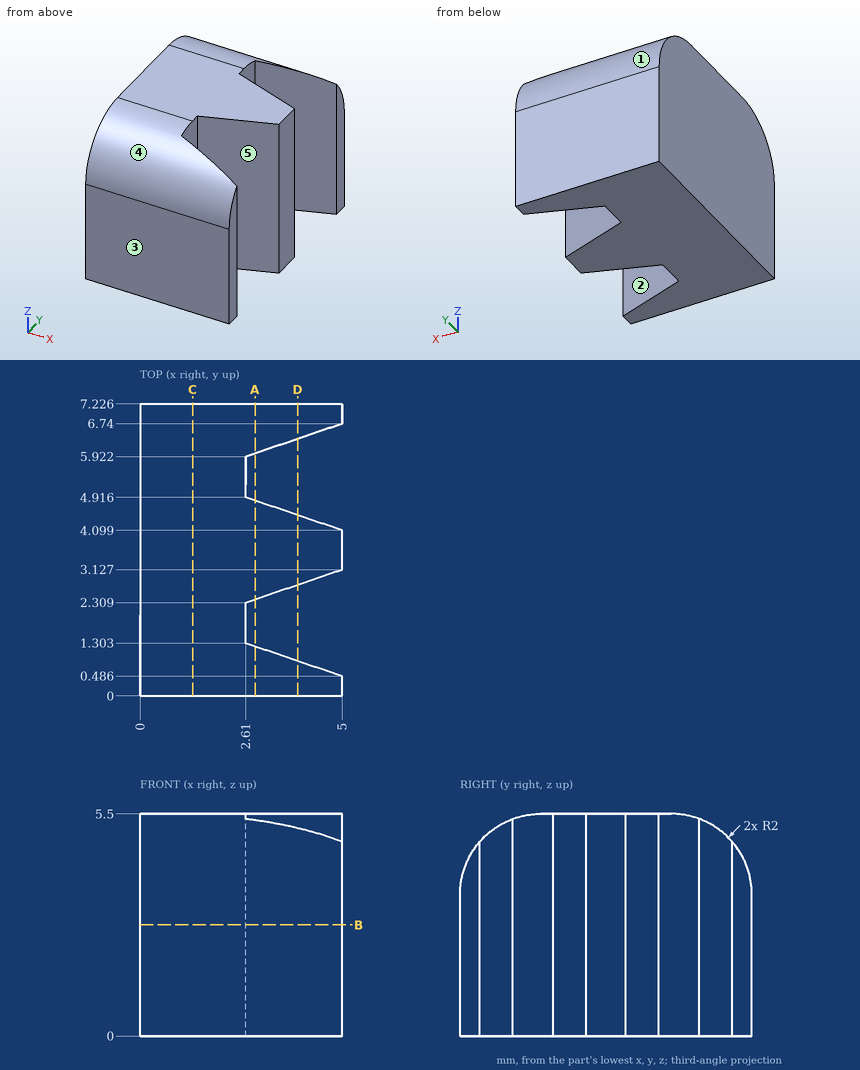
The figure shows three views and two pictorial views of one solid part (mm, origin at its lowest corner). Answer the questions. A direction names the side the tool comes from. Round coordinates to 2 decimals unless told otherwise and drop trailing zeros. Write each loop counter-clockwise with the first axis right and the second up, starting at its lowest first coordinate (ties: lowest second). Pieces come first, ordered by that corner, then holes. Notation, with made-up numbers: (-10, 43.25) - (-1, 43.25) arc R26 cw to (-1, 68.25) - close; hole circle Ø11 at (15, 36.5). An arc over 180 degrees is marked (long way). One line per question, with ' | ' between items. Start each with the question number.
1. Find the intervals of material crossed by probe 1 along Y at (x, z) = (4.2, 0.5) (1 decimal); probe 2 along Y at (x, z) = (2.75, 4) (1 decimal); probe 3 along Z at (x, y) = (1.75, 5.5), in increasing order. Write a range as [from, to].
2. Section C-C (x = 1.3) is taken. Determine the outline of the cut face in (y, z) (1 decimal), and give its area (3 significant figures).
3. For the marked faces 4 and 5, determine the directions among +Z, -Z, +X, -X, +Y, -Y from which every point of the face is accessible in a straight line to the end or side of a thin tool.
4. For a pull along Y with two mould halves and no side action, classify the marked faces 1, 2 and 3 as +Y half, -Y half, draft (parallel to the pull), parting line (faces both ways), or undercut.
5. Section D-D (x = 3.9) is taken. Give the number of separate pieces and of enclosed holes in the cut face, and give its area (3 significant figures).
6. Section A-A (x = 2.85) is taken. Determine the outline of the cut face in (y, z) (1 decimal).
7. Section B-B (z = 2.75) is taken. Determine the outline of the cut face in (x, y) (1 decimal), and give its area (3 significant figures).
8. Each of these flat-tipped pins is pushed along its axis until it touches: pin 1 (1.5 mm diameter, centred on x = 3.5, y = 5, fed in from +Z); pin 2 (1 mm diameter, centred on x = 2.5, y = 1, fed in from +Z). Where does it stop, or does it pass through?
Filled in:
1) probe 1: [0, 0.8], [2.9, 4.4], [6.5, 7.2] | probe 2: [0.1, 1.3], [2.4, 4.9], [6, 7.2] | probe 3: [0, 5.48]
2) outline: (0, 0) - (7.2, 0) - (7.2, 3.5) arc R2 ccw to (5.2, 5.5) - (2, 5.5) arc R2 ccw to (0, 3.5) - close | area: 38.0 mm²
3) face 4: +Z, +X, -X, -Y | face 5: +Z, -Z, +X
4) face 1: +Y half | face 2: undercut | face 3: -Y half
5) separate pieces: 3 | enclosed holes: 0 | area: 17.5 mm²
6) outline: (0, 0) - (1.2, 0) - (1.2, 5.3) arc R2 ccw to (0, 3.5) - close; (2.4, 0) - (4.8, 0) - (4.8, 5.5) - (2.4, 5.5) - close; (6, 0) - (7.2, 0) - (7.2, 3.5) arc R2 ccw to (6, 5.3) - close
7) outline: (0, 0) - (5, 0) - (5, 0.5) - (2.6, 1.3) - (2.6, 2.3) - (5, 3.1) - (5, 4.1) - (2.6, 4.9) - (2.6, 5.9) - (5, 6.7) - (5, 7.2) - (0, 7.2) - close | area: 27.4 mm²
8) pin 1: z = 5.5 | pin 2: z = 5.44
